Print and shaded views of the part. All mm, measured from the part's lowest x, y and z. Coordinates: 2 decimals unless noted, no trailing zeros. Order: outer loops, then holes, each group sorted by start corner. A loop starts at its lowest first (then second) coordinate and runs counter-clockwise, first axis right, second up.
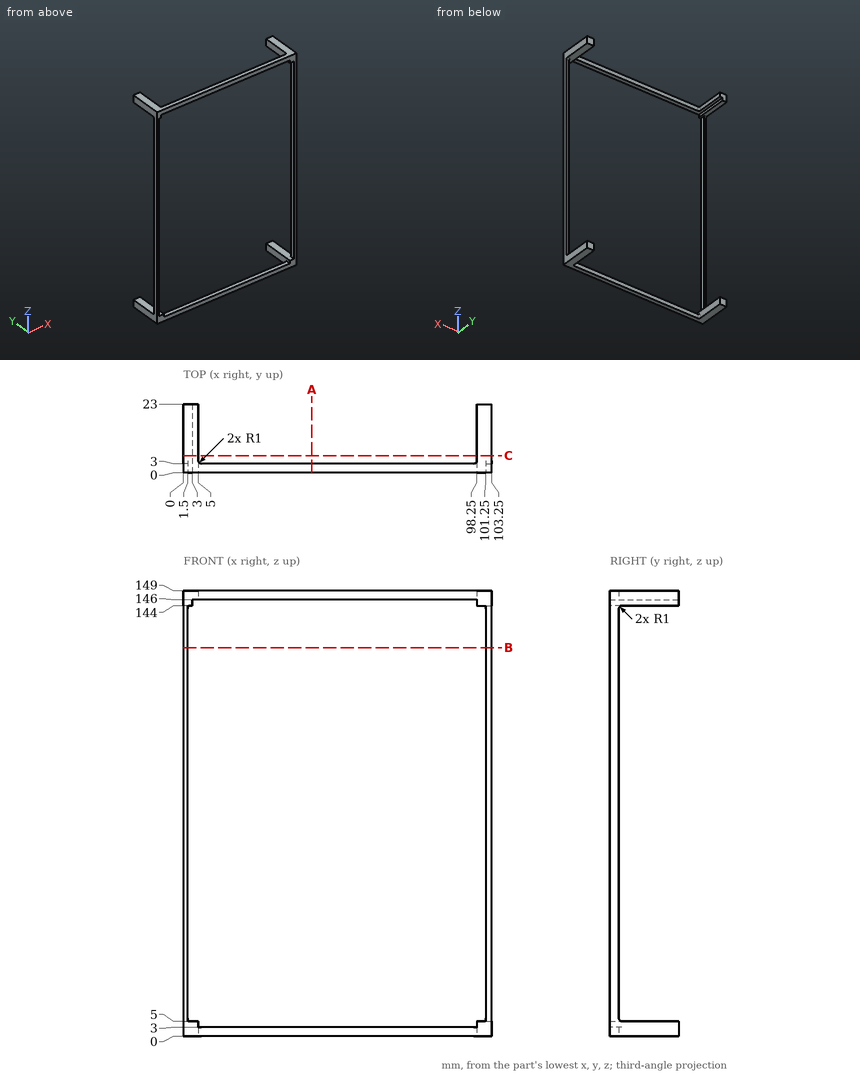
Q1. Drop flat-ended pins along their axis: P1, Ø0.9, axis at x = 50.5, z = 1.5, coming from the +Y side; P2, Ø12, axis at x = 45.5, y = 12.5, coming from the -Z side. Give the stop position or say it passes through.
Established:
P1: stops at y = 3
P2: passes through
Q2. Cut at B-B, the plane z = 130. List the corners of the cut face in (x, y).
Established:
outline: (0, 0) - (1.5, 0) - (1.5, 3) - (0, 3) - close; (101.25, 0) - (103.25, 0) - (103.25, 3) - (101.25, 3) - close
Q3. Cut at C-C, the plane y = 5.75. List the corners of the cut face in (x, z).
Established:
outline: (0, 0) - (5, 0) - (5, 5) - (0, 5) - close; (0, 144) - (3, 144) - (3, 146) - (5, 146) - (5, 149) - (0, 149) - close; (98.25, 0) - (103.25, 0) - (103.25, 5) - (98.25, 5) - close; (98.25, 144) - (103.25, 144) - (103.25, 149) - (98.25, 149) - close
Q4. Cut at A-A, the plane x = 43. List the corners of the cut face in (y, z).
Established:
outline: (0, 0) - (3, 0) - (3, 3) - (0, 3) - close; (0, 146) - (3, 146) - (3, 149) - (0, 149) - close
